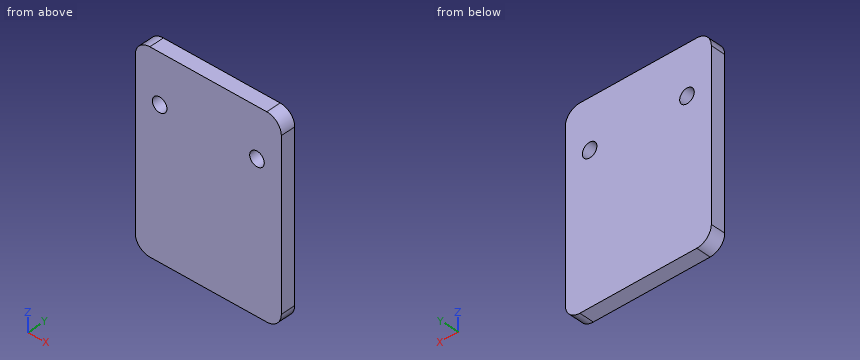
```python
from build123d import *

# Parameters (mm, degrees)
SKETCH_1_W          = 30
SKETCH_1_H          = 40
EXTRUDE_1_DEPTH     = 3
SKETCH_2_R          = 1.5
CUT_EXTRUDE_1_DEPTH = 26.179356624
FILLET_1_R          = 3


with BuildPart() as part:
    # 草图1 → 凸台-拉伸1 (new body)
    with BuildSketch(Plane(origin=(0, 0, 0), x_dir=(1, 0, 0), z_dir=(0, 1, 0))):
        Rectangle(SKETCH_1_W, SKETCH_1_H)
    extrude(amount=EXTRUDE_1_DEPTH)

    # 草图2 → 切除-拉伸1 (cut, through all)
    with BuildSketch(Plane(origin=(0, 3, 0), x_dir=(1, 0, 0), z_dir=(0, 1, 0))):
        with Locations(Location((-10, -10, 0), (0, 0, 270))):
            Circle(SKETCH_2_R)
        with Locations(Location((10, -10, 0), (0, 0, 90))):
            Circle(SKETCH_2_R)
    extrude(amount=-CUT_EXTRUDE_1_DEPTH, mode=Mode.SUBTRACT)

    # 圆角1
    fillet_1_edges = [part.edges().sort_by_distance(p)[0] for p in [
        (15, 1.5, 20),
        (-15, 1.5, 20),
        (-15, 1.5, -20),
        (15, 1.5, -20),
    ]]
    fillet(fillet_1_edges, radius=FILLET_1_R)


solid = part.part
```
For this review, take the finished solid that the model builds, in its own axes (mm). Give positions to 0.01 mm unless a question says otherwise; leave off trailing zeros. Write each loop counter-clockwise with the first axis right and the second up, starting at its lowest first coordinate (ties: lowest second). Pieces come first, ordered by that corner, then holes. Notation, with made-up numbers: M 6,12 L 57,12 A8 ccw 57,16 Z; hole C 81,20.5 d1. An arc over 180 degrees is marked long. Answer as a JSON object with one key per item and string values. Group by question number.
Item 1: Consider section A-A on z = 10. Write out the cut boundary in (x, y), plus the area to 3 significant figures.
Item 2: Consider section C-C on y = 1.1. Write out the cut boundary in (x, z), plus the area to 3 significant figures.
Item 3: Consider section B-B on x = 10. Write out the cut boundary in (y, z).
Item 4: For probe 1 along X at (y, z) = (0.8, 10); probe 2 along Z at (x, y) = (10, 1.45); probe 3 along X at (y, z) = (2.8, 9), list the stretches that pass through material, from the lowest coordinate up. Write a range as [from, to].
Check result:
{
 "1": {"outline": "M -15,0 L -11.5,0 L -11.5,3 L -15,3 Z; M -8.5,0 L 8.5,0 L 8.5,3 L -8.5,3 Z; M 11.5,0 L 15,0 L 15,3 L 11.5,3 Z", "area": "72.0 mm^2"},
 "2": {"outline": "M -15,-17 A3 ccw -12,-20 L 12,-20 A3 ccw 15,-17 L 15,17 A3 ccw 12,20 L -12,20 A3 ccw -15,17 Z; hole C -10,10 d3; hole C 10,10 d3", "area": "1,180 mm^2"},
 "3": {"outline": "M 0,-20 L 3,-20 L 3,8.5 L 0,8.5 Z; M 0,11.5 L 3,11.5 L 3,20 L 0,20 Z"},
 "4": {"probe 1": "x = [-15, -11.5], [-8.5, 8.5], [11.5, 15]", "probe 2": "z = [-20, 8.5], [11.5, 20]", "probe 3": "x = [-15, -11.12], [-8.88, 8.88], [11.12, 15]"}
}
